Can you work these out from the drawing? Everything is in mm from the part's minimum corner. Give positions to 0.01 mm unless a question says otherwise; leave off trailing zeros. Write each loop counter-clockwise with the first axis right and the second up, starting at its lowest first coordinate (ties: lowest second). Pieces come first, ordered by that corner, then holes. Notation, with made-up numbers: M 77,5.5 L 112,5.5 A21 cw 112,22.5 Z; hole C 50,-34.75 d11. An arc over 180 degrees is marked long. One line per item, written item: value.
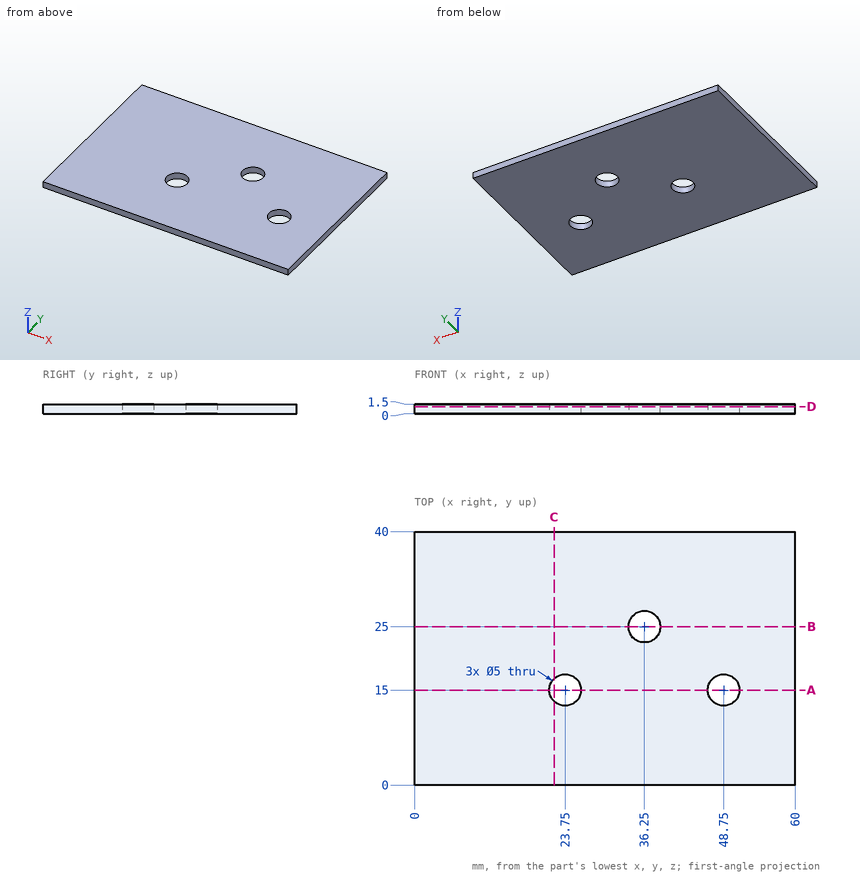
1) If we section it at C-C, the plane x = 22: Write out the boundary of the cut face in (y, z).
Outcome:
outline: M 0,0 L 13.21,0 L 13.21,1.5 L 0,1.5 Z; M 16.79,0 L 40,0 L 40,1.5 L 16.79,1.5 Z
2) If we section it at A-A, the plane y = 15: Write out the boundary of the cut face in (x, z), then the cut area to 3 significant figures.
Outcome:
outline: M 0,0 L 21.25,0 L 21.25,1.5 L 0,1.5 Z; M 26.25,0 L 46.25,0 L 46.25,1.5 L 26.25,1.5 Z; M 51.25,0 L 60,0 L 60,1.5 L 51.25,1.5 Z
area: 75.0 mm^2
3) If we section it at B-B, the plane y = 25: Write out the boundary of the cut face in (x, z), then the cut area to 3 significant figures.
Outcome:
outline: M 0,0 L 33.75,0 L 33.75,1.5 L 0,1.5 Z; M 38.75,0 L 60,0 L 60,1.5 L 38.75,1.5 Z
area: 82.5 mm^2
4) Please list where these lines run through material, in increasing order: L1, parallel to X at y = 15, z = 0.6; L2, parallel to X at y = 25, z = 0.95; L3, parallel to Y at x = 49, z = 0.4. Write a range as from..to.
Outcome:
L1: x = 0..21.25, 26.25..46.25, 51.25..60
L2: x = 0..33.75, 38.75..60
L3: y = 0..12.51, 17.49..40
5) If we section it at D-D, the plane z = 1.1: Write out the boundary of the cut face in (x, y), then the cut area to 3 significant figures.
Outcome:
outline: M 0,0 L 60,0 L 60,40 L 0,40 Z; hole C 23.75,15 d5; hole C 36.25,25 d5; hole C 48.75,15 d5
area: 2,340 mm^2
